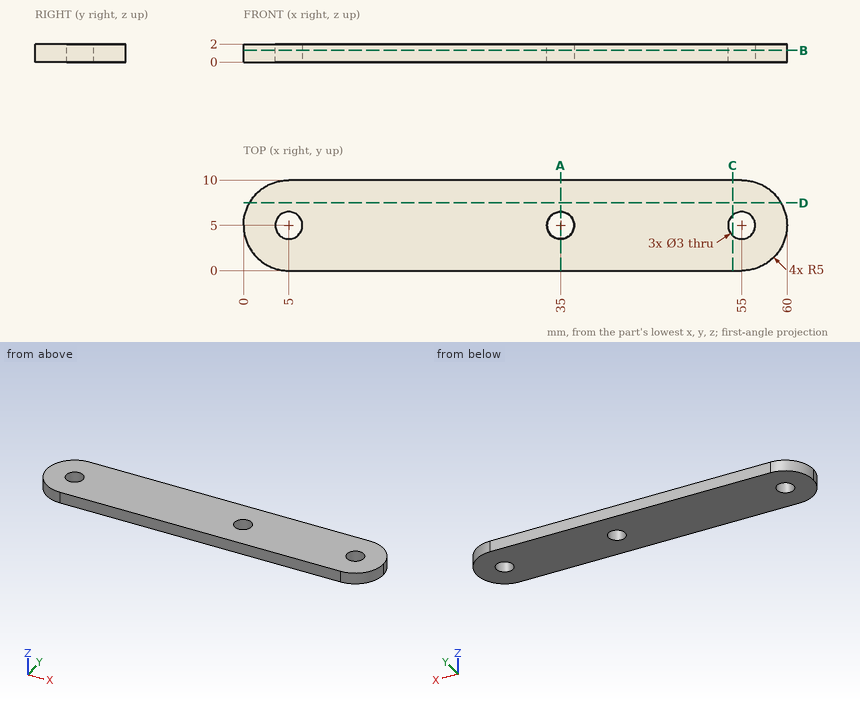
Verification items for this drawing (mm, ordinates from the low corner). Give positions to 0.01 mm unless a question says otherwise; leave off trailing zeros. Loops run counter-clockwise (first coordinate to the right, second up) from the corner with the lowest first, then second, coordinate; pieces in that order, holes last. Notation, with made-up numbers: M 2.5,76.25 L 16.5,76.25 A24 ccw 16.5,111.25 Z; hole C 83,38.25 d1. An arc over 180 degrees is marked long. Answer in a Markdown table with one row per item.
1) Thickness scan on line 1 (Y direction, x = 35, z = 0.5); line 2 (X direction, y = 4.75, z = 0.95); line 3 (X direction, y = 0.75, z = 0.9). Record the ranges inside material, lowest first.
Solutions:
| item | result |
|---|---|
| line 1 | y = 0 to 3.5, 6.5 to 10 |
| line 2 | x = 0.01 to 3.52, 6.48 to 33.52, 36.48 to 53.52, 56.48 to 59.99 |
| line 3 | x = 2.37 to 57.63 |
2) Cross-section at D-D (y = 7.5). Enter the section's corners in (x, z).
Solutions:
| item | result |
|---|---|
| outline | M 0.67,0 L 59.33,0 L 59.33,2 L 0.67,2 Z |
3) Cross-section at B-B (z = 1.3). Count the separate pieces of the cut face and the enclosed holes in it, plus the area to 3 significant figures.
Solutions:
| item | result |
|---|---|
| separate pieces | 1 |
| enclosed holes | 3 |
| area | 557 mm^2 |
4) Cross-section at A-A (x = 35). Enter the section's corners in (y, z), plus the area to 3 significant figures.
Solutions:
| item | result |
|---|---|
| outline | M 0,0 L 3.5,0 L 3.5,2 L 0,2 Z; M 6.5,0 L 10,0 L 10,2 L 6.5,2 Z |
| area | 14.0 mm^2 |
5) Cross-section at C-C (x = 54). Enter the section's corners in (y, z).
Solutions:
| item | result |
|---|---|
| outline | M 0,0 L 3.88,0 L 3.88,2 L 0,2 Z; M 6.12,0 L 10,0 L 10,2 L 6.12,2 Z |
